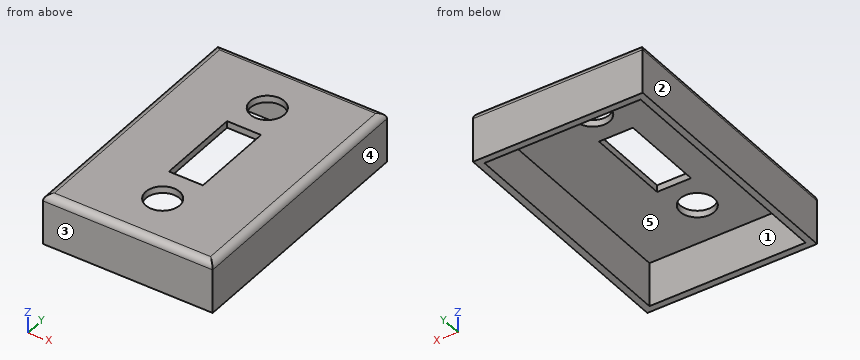
```python
from build123d import *

# Parameters (mm, degrees)
SKETCH1_W           = 50
SKETCH1_H           = 75
BOSS_EXTRUDE1_DEPTH = 15
SHELL3_T            = -2
FILLET1_R           = 2
SKETCH2_R           = 5
SKETCH2_W           = 10
SKETCH2_H           = 25
CUT_EXTRUDE1_DEPTH  = 16


with BuildPart() as part:
    # Sketch1 → Boss-Extrude1 (new body)
    with BuildSketch(Plane.XY):
        with Locations((25, 37.5)):
            Rectangle(SKETCH1_W, SKETCH1_H)
    extrude(amount=BOSS_EXTRUDE1_DEPTH)

    # Shell3
    shell3_openings = [part.faces().sort_by_distance(p)[0] for p in [
        (25, 37.5, 0),
    ]]
    offset(amount=SHELL3_T, openings=shell3_openings, kind=Kind.INTERSECTION)

    # Fillet1
    fillet1_edges = [part.edges().sort_by_distance(p)[0] for p in [
        (50, 37.5, 15),
        (25, 75, 15),
        (0, 37.5, 15),
        (25, 0, 15),
    ]]
    fillet(fillet1_edges, radius=FILLET1_R)

    # Sketch2 → Cut-Extrude1 (cut, through all)
    with BuildSketch(Plane.XY.offset(15)):
        with Locations((25, 60)):
            Circle(SKETCH2_R)
        with Locations((25, 15)):
            Circle(SKETCH2_R)
        with Locations((25, 37.5)):
            Rectangle(SKETCH2_W, SKETCH2_H)
    extrude(amount=-CUT_EXTRUDE1_DEPTH, mode=Mode.SUBTRACT)


solid = part.part
```
Part model, mm, in its own coordinate system. Face numbers are marked on the shaded views. A direction names the side the tool comes from. Coordinates: 2 decimals unless noted, no trailing zeros. Order: outer loops, then holes, each group sorted by start corner. A loop starts at its lowest first (then second) coordinate and runs counter-clockwise, first axis right, second up. Notation, with made-up numbers: (24.25, 27) -> (76.25, 27) arc R22 cw to (76.25, 50) -> close; hole circle Ø3 at (5.25, -13). An arc over 180 degrees is marked (long way). Put each result on its own line as item: value. Start each with the question number.
(1) Band-saw the part on D-D (x = 38). Give the cut face in (y, z), then the cut area to 3 significant figures.
(2) Pin check, flat tips, straight feed: pin 1 Ø2 at (y, z) = (34, 14.5) entering from -X; pin 2 Ø11.5 at (x, y) = (25, 60) entering from -Z; pin 3 Ø0.6 at (x, z) = (24, 14) entering from -Y. Stop position of each tip, or through.
(3) Band-saw the part on C-C (y = 15). Give the cut face in (x, z).
(4) Probe line 1 along X through (y, z) = (23, 12); line 2 along Y through (x, z) = (5, 7.5); line 3 along Y through (x, z) = (25, 13.8). List the from-to ranges inside material, lowest first. Write a range as [from, to].
(5) Band-saw the part on B-B (z = 4). Give the cut face in (x, y).
(6) Mould opens along X. For the marked faces 1, 2 and 3 say: pulls with the +X half, pulls with the -X half, needs draft (parallel to the pull), parting line crosses it, or undercut.
(7) Band-saw the part on A-A (x = 25). Give the cut face in (y, z), then the cut area to 3 significant figures.
(8) Which spindle directions (+Z, -Z, +X, -X, +Y, -Y) get a long thin tool onto all of the face, cutting with end or side? Do the marked faces 4 and 5. Say none if no direction does.
Determined:
1. outline: (0, 0) -> (2, 0) -> (2, 13) -> (73, 13) -> (73, 0) -> (75, 0) -> (75, 13) arc R2 ccw to (73, 15) -> (2, 15) arc R2 ccw to (0, 13) -> close
1. area: 200 mm²
2. pin 1: stops at x = 0.06
2. pin 2: stops at z = 13
2. pin 3: stops at y = 0.13
3. outline: (0, 0) -> (2, 0) -> (2, 13) -> (20, 13) -> (20, 15) -> (2, 15) arc R2 ccw to (0, 13) -> close; (30, 13) -> (48, 13) -> (48, 0) -> (50, 0) -> (50, 13) arc R2 ccw to (48, 15) -> (30, 15) -> close
4. line 1: x = [0, 2], [48, 50]
4. line 2: y = [0, 2], [73, 75]
4. line 3: y = [0.17, 10], [20, 25], [50, 55], [65, 74.83]
5. outline: (0, 0) -> (50, 0) -> (50, 75) -> (0, 75) -> close; hole (2, 2) -> (48, 2) -> (48, 73) -> (2, 73) -> close
6. face 1: undercut
6. face 2: pulls with the -X half
6. face 3: needs draft
7. outline: (0, 0) -> (2, 0) -> (2, 13) -> (10, 13) -> (10, 15) -> (2, 15) arc R2 ccw to (0, 13) -> close; (20, 13) -> (25, 13) -> (25, 15) -> (20, 15) -> close; (50, 13) -> (55, 13) -> (55, 15) -> (50, 15) -> close; (65, 13) -> (73, 13) -> (73, 0) -> (75, 0) -> (75, 13) arc R2 ccw to (73, 15) -> (65, 15) -> close
7. area: 110 mm²
8. face 4: +Z, -Z, +X, +Y, -Y
8. face 5: -Z
